```python
from build123d import *
from OCP.BRepFilletAPI import BRepFilletAPI_MakeFillet

# Parameters (mm, degrees)
DODANIE_WYCI_GNI_CIE1_DEPTH = 27
WYTNIJ_WYCI_GNI_CIE1_REACH  = 71.794
SZKIC2_R                    = 0.55
WYTNIJ_WYCI_GNI_CIE2_START  = -7.5
SZKIC2_3_R                  = 4.3
SZKIC2_3_R_2                = 2.05
WYTNIJ_WYCI_GNI_CIE2_DEPTH  = 2
WYTNIJ_WYCI_GNI_CIE3_REACH  = 68.633
ZAOKR_GLENIE1_R             = 1
ZAOKR_GLENIE2_R1            = 8
ZAOKR_GLENIE2_R2            = 4
OTW_R_POD_RUB_M41_D         = 4.3


with BuildPart() as part:
    # Szkic1 → Dodanie-wyciągnięcie1 (new body)
    with BuildSketch(Plane(origin=(0, 0, 0), x_dir=(0, 0, -1), z_dir=(1, 0, 0))):
        Polygon((-20.551283841, -19.152030835), (-39.051283841, -19.152030835), (-39.051283841, -16.652030835), (-23.109904513, -16.652030835), (-23.109904513, -14.652030835), (-50.551283841, -14.652030835), (-50.551283841, 10.347969165), (-55.551283841, 10.347969165), (-55.551283841, -22.152030835), (-20.551283841, -22.152030835), align=None)
    extrude(amount=-DODANIE_WYCI_GNI_CIE1_DEPTH)

    # Szkic2 → Wytnij-wyciągnięcie1 (cut, up to next)
    with BuildSketch(Plane.XZ.offset(22.152030835), mode=Mode.PRIVATE) as wytnij_wyci_gni_cie1_sk1:
        with Locations(Location((-3, 23.051283841, 0), (0, 0, 270))):
            Circle(SZKIC2_R)
    wytnij_wyci_gni_cie1_tool1 = extrude(wytnij_wyci_gni_cie1_sk1.sketch, amount=-WYTNIJ_WYCI_GNI_CIE1_REACH, mode=Mode.PRIVATE) & part.part
    # Szkic2 → Wytnij-wyciągnięcie1 (cut, up to next)
    with BuildSketch(Plane.XZ.offset(22.152030835), mode=Mode.PRIVATE) as wytnij_wyci_gni_cie1_sk2:
        with Locations(Location((-3, 35.551283841, 0), (0, 0, 270))):
            Circle(SZKIC2_R)
    wytnij_wyci_gni_cie1_tool2 = extrude(wytnij_wyci_gni_cie1_sk2.sketch, amount=-WYTNIJ_WYCI_GNI_CIE1_REACH, mode=Mode.PRIVATE) & part.part
    # Szkic2 → Wytnij-wyciągnięcie1 (cut, up to next)
    with BuildSketch(Plane.XZ.offset(22.152030835), mode=Mode.PRIVATE) as wytnij_wyci_gni_cie1_sk3:
        with Locations(Location((-24, 35.551283841, 0), (0, 0, 270))):
            Circle(SZKIC2_R)
    wytnij_wyci_gni_cie1_tool3 = extrude(wytnij_wyci_gni_cie1_sk3.sketch, amount=-WYTNIJ_WYCI_GNI_CIE1_REACH, mode=Mode.PRIVATE) & part.part
    # Szkic2 → Wytnij-wyciągnięcie1 (cut, up to next)
    with BuildSketch(Plane.XZ.offset(22.152030835), mode=Mode.PRIVATE) as wytnij_wyci_gni_cie1_sk4:
        with Locations(Location((-24, 23.051283841, 0), (0, 0, 270))):
            Circle(SZKIC2_R)
    wytnij_wyci_gni_cie1_tool4 = extrude(wytnij_wyci_gni_cie1_sk4.sketch, amount=-WYTNIJ_WYCI_GNI_CIE1_REACH, mode=Mode.PRIVATE) & part.part
    add(wytnij_wyci_gni_cie1_tool1.solids().sort_by_distance((-3, -22.152031, 23.051284))[0], mode=Mode.SUBTRACT)
    add(wytnij_wyci_gni_cie1_tool2.solids().sort_by_distance((-3, -22.152031, 35.551284))[0], mode=Mode.SUBTRACT)
    add(wytnij_wyci_gni_cie1_tool3.solids().sort_by_distance((-24, -22.152031, 35.551284))[0], mode=Mode.SUBTRACT)
    add(wytnij_wyci_gni_cie1_tool4.solids().sort_by_distance((-24, -22.152031, 23.051284))[0], mode=Mode.SUBTRACT)

    # Szkic2<3> → Wytnij-wyciągnięcie2 (cut)
    with BuildSketch(Plane.XZ.offset(22.152030835).offset(WYTNIJ_WYCI_GNI_CIE2_START)):
        with Locations((-13.468476265, 23.109904513)):
            Circle(SZKIC2_3_R)
        with Locations((-3, 23.051283841)):
            Circle(SZKIC2_3_R_2)
        with Locations((-24, 23.051283841)):
            Circle(SZKIC2_3_R_2)
        with Locations(Location((-24, 35.551283841, 0), (0, 0, 270))):
            Circle(SZKIC2_3_R_2)
        with Locations(Location((-3, 35.551283841, 0), (0, 0, 270))):
            Circle(SZKIC2_3_R_2)
    extrude(amount=WYTNIJ_WYCI_GNI_CIE2_DEPTH, mode=Mode.SUBTRACT)

    # Szkic3 → Wytnij-wyciągnięcie3 (cut, up to next)
    with BuildSketch(Plane(origin=(0, -14.652030835, 0), x_dir=(1, 0, 0), z_dir=(0, 1, 0)), mode=Mode.PRIVATE) as wytnij_wyci_gni_cie3_sk1:
        with BuildLine():
            ThreePointArc((-24, -37.601283841), (-26.05, -35.551283841), (-24, -33.501283841))
            Line((-24, -33.501283841), (-27, -33.501283841))
            Line((-27, -33.501283841), (-27, -37.601283841))
            Line((-27, -37.601283841), (-24, -37.601283841))
        make_face()
    wytnij_wyci_gni_cie3_tool1 = extrude(wytnij_wyci_gni_cie3_sk1.sketch, amount=-WYTNIJ_WYCI_GNI_CIE3_REACH, mode=Mode.PRIVATE) & part.part
    # Szkic3 → Wytnij-wyciągnięcie3 (cut, up to next)
    with BuildSketch(Plane(origin=(0, -14.652030835, 0), x_dir=(1, 0, 0), z_dir=(0, 1, 0)), mode=Mode.PRIVATE) as wytnij_wyci_gni_cie3_sk2:
        with BuildLine():
            Line((-27, -23.109904513), (-27, -25.101283841))
            Line((-27, -25.101283841), (-24, -25.101283841))
            ThreePointArc((-24, -25.101283841), (-25.428693043, -24.521432197), (-26.049161686, -23.109904513))
            Line((-26.049161686, -23.109904513), (-27, -23.109904513))
        make_face()
    wytnij_wyci_gni_cie3_tool2 = extrude(wytnij_wyci_gni_cie3_sk2.sketch, amount=-WYTNIJ_WYCI_GNI_CIE3_REACH, mode=Mode.PRIVATE) & part.part
    # Szkic3 → Wytnij-wyciągnięcie3 (cut, up to next)
    with BuildSketch(Plane(origin=(0, -14.652030835, 0), x_dir=(1, 0, 0), z_dir=(0, 1, 0)), mode=Mode.PRIVATE) as wytnij_wyci_gni_cie3_sk3:
        with BuildLine():
            Line((-3, -25.101283841), (0, -25.101283841))
            Line((0, -25.101283841), (0, -23.109904513))
            Line((0, -23.109904513), (-0.950838314, -23.109904513))
            ThreePointArc((-0.950838314, -23.109904513), (-1.571306957, -24.521432197), (-3, -25.101283841))
        make_face()
    wytnij_wyci_gni_cie3_tool3 = extrude(wytnij_wyci_gni_cie3_sk3.sketch, amount=-WYTNIJ_WYCI_GNI_CIE3_REACH, mode=Mode.PRIVATE) & part.part
    # Szkic3 → Wytnij-wyciągnięcie3 (cut, up to next)
    with BuildSketch(Plane(origin=(0, -14.652030835, 0), x_dir=(1, 0, 0), z_dir=(0, 1, 0)), mode=Mode.PRIVATE) as wytnij_wyci_gni_cie3_sk4:
        with BuildLine():
            Line((0, -33.501283841), (-3, -33.501283841))
            ThreePointArc((-3, -33.501283841), (-1.550431099, -34.101714939), (-0.95, -35.551283841))
            ThreePointArc((-0.95, -35.551283841), (-1.550431099, -37.000852742), (-3, -37.601283841))
            Line((-3, -37.601283841), (0, -37.601283841))
            Line((0, -37.601283841), (0, -33.501283841))
        make_face()
    wytnij_wyci_gni_cie3_tool4 = extrude(wytnij_wyci_gni_cie3_sk4.sketch, amount=-WYTNIJ_WYCI_GNI_CIE3_REACH, mode=Mode.PRIVATE) & part.part
    add(wytnij_wyci_gni_cie3_tool1.solids().sort_by_distance((-26.229723, -14.652031, 35.551284))[0], mode=Mode.SUBTRACT)
    add(wytnij_wyci_gni_cie3_tool2.solids().sort_by_distance((-26.223837, -14.652031, 24.279211))[0], mode=Mode.SUBTRACT)
    add(wytnij_wyci_gni_cie3_tool3.solids().sort_by_distance((-0.776163, -14.652031, 24.279211))[0], mode=Mode.SUBTRACT)
    add(wytnij_wyci_gni_cie3_tool4.solids().sort_by_distance((-0.770277, -14.652031, 35.551284))[0], mode=Mode.SUBTRACT)

    # Zaokrąglenie1
    zaokr_glenie1_edges = [part.edges().sort_by_distance(p)[0] for p in [
        (-27, -15.652030835, 25.101283841),
        (-27, -15.652030835, 33.501283841),
        (-27, -15.652030835, 37.601283841),
        (-5.049161686, -15.652030835, 23.109904513),
        (-21.950838314, -15.652030835, 23.109904513),
        (-9.168476265, -15.652030835, 23.109904513),
        (-17.768476265, -15.652030835, 23.109904513),
        (0, -15.652030835, 33.501283841),
        (0, -15.652030835, 37.601283841),
        (0, -15.652030835, 25.101283841),
    ]]
    fillet(zaokr_glenie1_edges, radius=ZAOKR_GLENIE1_R)

    # Zaokrąglenie2: one fillet with a radius per group of edges: ONE call of the kernel's fillet builder (fillet() takes one radius for all edges)
    zaokr_glenie2_edges_1 = [part.edges().sort_by_distance(p)[0] for p in [
        (-13.5, -22.152030835, 55.551283841),
    ]]
    zaokr_glenie2_edges_2 = [part.edges().sort_by_distance(p)[0] for p in [
        (-13.5, -14.652030835, 50.551283841),
    ]]
    zaokr_glenie2 = BRepFilletAPI_MakeFillet(part.part.solid().wrapped)
    for e in zaokr_glenie2_edges_1:
        zaokr_glenie2.Add(ZAOKR_GLENIE2_R1, e.wrapped)
    for e in zaokr_glenie2_edges_2:
        zaokr_glenie2.Add(ZAOKR_GLENIE2_R2, e.wrapped)
    add(Compound.cast(zaokr_glenie2.Shape()), mode=Mode.REPLACE)

    # Otwór pod śrubę M41 (through all)
    with Locations(Plane(origin=(0, 0, 50.551283841), x_dir=(-1, 0, 0), z_dir=(0, 0, -1))):
        with Locations((22, -2.152030835), (13.5, -2.152030835), (5, -2.152030835), (5, 6.347969165), (13.5, 6.347969165), (22, 6.347969165)):
            Hole(OTW_R_POD_RUB_M41_D / 2)


solid = part.part
```
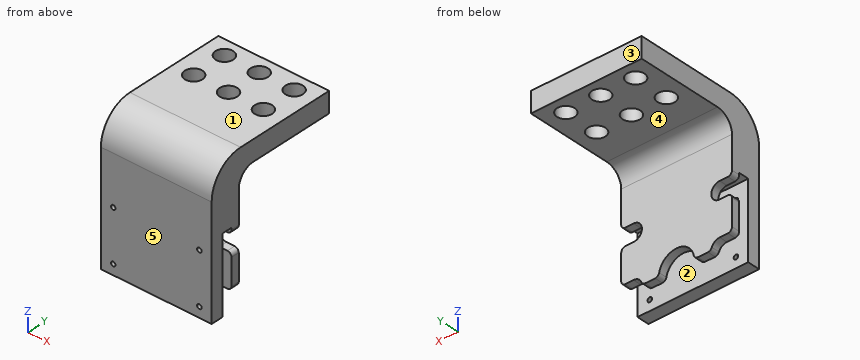
Input: part model. Units: mm. Frame: model coordinates. Face numbers are marked on the shaded views. A direction names the side the tool comes from. Coordinates: 2 decimals unless noted, no trailing zeros. Loops run counter-clockwise (first coordinate to the right, second up) from the corner with the lowest first, then second, coordinate; pieces in that order, holes last.
Q1. Section D-D, the plane y = 1. Return the cut outline in (x, z).
Results are:
outline: (-27, 50.55) - (0, 50.55) - (0, 55.55) - (-27, 55.55) - close
Q2. Section B-B, the plane x = -13.5. Return the cut outline in (y, z).
Results are:
outline: (-22.15, 20.55) - (-19.15, 20.55) - (-19.15, 39.05) - (-16.65, 39.05) - (-16.65, 27.41) - (-14.65, 27.41) - (-14.65, 46.55) arc R4 cw to (-10.65, 50.55) - (-4.3, 50.55) - (-4.3, 55.55) - (-14.15, 55.55) arc R8 ccw to (-22.15, 47.55) - close; (0, 50.55) - (4.2, 50.55) - (4.2, 55.55) - (0, 55.55) - close; (8.5, 50.55) - (10.35, 50.55) - (10.35, 55.55) - (8.5, 55.55) - close
Q3. Mould query, pull axis Y, two halves, no side actions, for the marked faces 1, 2 and 3. Classes: +Y half, -Y half, draft (parallel to the pull), parting line (faces both ways), or undercut.
Results are:
face 1: draft
face 2: undercut
face 3: +Y half
Q4. Set-up query: the marked faces 4 and 5. Return all of +Z, -Z, +X, -X, +Y, -Y with unobstructed straight access to the full face (end or side cutting, diameter ignored); none if empty.
Results are:
face 4: -Z, +X, -X, +Y
face 5: +Z, -Z, +X, -X, -Y
Q5. Contact query for flat-ended pins moving along their axis: pin 1 (1.6 mm diameter, centred on x = -25.5, y = -15.5, fed in from +Z); pin 2 (1.6 mm diameter, centred on x = -25.5, y = -15.5, fed in from -Z); pin 3 (5.5 mm diameter, centred on x = -22, y = 6.35, fed in from -Z). Output: stop coordinate, or through.
Results are:
pin 1: stops at z = 55.53
pin 2: stops at z = 25.1
pin 3: stops at z = 50.55
Q6. Section A-A, the plane z = 37. Return the cut outline in (x, y).
Results are:
outline: (-27, -22.15) - (0, -22.15) - (0, -19.15) - (-27, -19.15) - close; (-22.55, -16.65) - (-4.45, -16.65) - (-4.45, -14.65) - (-22.55, -14.65) - close
Q7. Section C-C, the plane z = 45. Return the cut outline in (x, y).
Results are:
outline: (-27, -22.15) - (0, -22.15) - (0, -14.65) - (-27, -14.65) - close
Q8. Line query: line 1 along Y through (x, z) = (-2.25, 26.5); line 2 along Y through (x, z) = (-13.5, 53); line 3 along Y through (x, z) = (-5, 52.5). Output: solid intervals per line, ascending.
Results are:
line 1: y = -22.15 to -19.15, -16.65 to -14.65
line 2: y = -20.01 to -4.3, 0 to 4.2, 8.5 to 10.35
line 3: y = -20.44 to -4.3, 0 to 4.2, 8.5 to 10.35
